from build123d import *

# Parameters (mm, degrees)
SKETCH_2_W          = 26.5
SKETCH_2_H          = 14.5
EXTRUDE_1_DEPTH     = 57
SKETCH_6_W          = 22.5
SKETCH_6_H          = 10.5
CUT_EXTRUDE_1_DEPTH = 49
SKETCH_7_W          = 26.5
SKETCH_7_H          = 16
EXTRUDE_2_DEPTH     = 24.8
FILLET_1_R          = 5
FILLET_2_R          = 1
FILLET_4_R          = 1
FILLET_5_R          = 1
FILLET_6_R          = 1
CUT_EXTRUDE_2_DEPTH = 20
SKETCH_10_W         = 10
SKETCH_10_H         = 3.5
CUT_EXTRUDE_3_DEPTH = 40


with BuildPart() as part:
    # ｽｹｯﾁ2 → ﾎﾞｽ - 押し出し1 (new body)
    with BuildSketch(Plane.XY):
        with Locations((13.25, 7.25)):
            Rectangle(SKETCH_2_W, SKETCH_2_H)
    extrude(amount=EXTRUDE_1_DEPTH)

    # ｽｹｯﾁ6 → ｶｯﾄ - 押し出し1 (cut)
    with BuildSketch(Plane.XY.offset(57)):
        with Locations((13.25, 7.25)):
            Rectangle(SKETCH_6_W, SKETCH_6_H)
    extrude(amount=-CUT_EXTRUDE_1_DEPTH, mode=Mode.SUBTRACT)

    # ｽｹｯﾁ7 → ﾎﾞｽ - 押し出し2 (add)
    with BuildSketch(Plane.XZ):
        with Locations((13.25, 8)):
            Rectangle(SKETCH_7_W, SKETCH_7_H)
    extrude(amount=EXTRUDE_2_DEPTH)

    # ﾌｨﾚｯﾄ1
    fillet_1_edges = [part.edges().sort_by_distance(p)[0] for p in [
        (13.25, 0, 16),
    ]]
    fillet(fillet_1_edges, radius=FILLET_1_R)

    # ﾌｨﾚｯﾄ2
    fillet_2_edges = [part.edges().sort_by_distance(p)[0] for p in [
        (26.5, 14.5, 28.5),
    ]]
    fillet(fillet_2_edges, radius=FILLET_2_R)

    # ﾌｨﾚｯﾄ4
    fillet_4_edges = [part.edges().sort_by_distance(p)[0] for p in [
        (26.5, -14.9, 16),
        (26.5, -24.8, 8),
        (26.5, -1.464466094, 17.464466094),
        (12.75, 14.5, 0),
        (26.207106781, 14.207106781, 0),
        (26.5, -5.65, 0),
        (26.5, 0, 39),
    ]]
    fillet(fillet_4_edges, radius=FILLET_4_R)

    # ﾌｨﾚｯﾄ5
    # the kernel refuses this fillet: 1 mm, written as the material it takes off along each edge
    with BuildSketch(Plane(origin=(25.5, -23.8, 15), x_dir=(0, -1, 0), z_dir=(0, 0, 1))) as fillet_5_piece_1_section:
        Polygon((0, 0), (FILLET_5_R, 0), (FILLET_5_R, FILLET_5_R), (0, FILLET_5_R), align=None)
    fillet_5_piece_1 = extrude(amount=FILLET_5_R, mode=Mode.PRIVATE)
    fillet_5_piece_1 = fillet_5_piece_1 - Plane(origin=(25.5, -23.8, 15), x_dir=(-0.7071067811865475, 0.7071067811865475, 0), z_dir=(0, 0, 1)) * Sphere(FILLET_5_R, mode=Mode.PRIVATE)
    add(fillet_5_piece_1, mode=Mode.SUBTRACT)
    with BuildSketch(Plane(origin=(25.5, -23.8, 1), x_dir=(0, -1, 0), z_dir=(0, 0, -1))) as fillet_5_piece_2_section:
        Polygon((0, 0), (FILLET_5_R, 0), (FILLET_5_R, -FILLET_5_R), (0, -FILLET_5_R), align=None)
    fillet_5_piece_2 = extrude(amount=FILLET_5_R, mode=Mode.PRIVATE)
    fillet_5_piece_2 = fillet_5_piece_2 - Plane(origin=(25.5, -23.8, 1), x_dir=(-0.7071067811865475, 0.7071067811865475, 0), z_dir=(0, 0, -1)) * Sphere(FILLET_5_R, mode=Mode.PRIVATE)
    add(fillet_5_piece_2, mode=Mode.SUBTRACT)
    with BuildSketch(Plane(origin=(1, -23.8, 15), x_dir=(-1, 0, 0), z_dir=(0, -1, 0))) as fillet_5_piece_3_section:
        Polygon((0, 0), (FILLET_5_R, 0), (FILLET_5_R, -FILLET_5_R), (0, -FILLET_5_R), align=None)
    fillet_5_piece_3 = extrude(amount=FILLET_5_R, mode=Mode.PRIVATE)
    fillet_5_piece_3 = fillet_5_piece_3 - Plane(origin=(1, -23.8, 15), x_dir=(0.7071067811865475, 0, -0.7071067811865475), z_dir=(0, -1, 0)) * Sphere(FILLET_5_R, mode=Mode.PRIVATE)
    add(fillet_5_piece_3, mode=Mode.SUBTRACT)
    with BuildSketch(Plane(origin=(1, -23.8, 1), x_dir=(-1, 0, 0), z_dir=(0, 0, -1))) as fillet_5_piece_4_section:
        Polygon((0, 0), (FILLET_5_R, 0), (FILLET_5_R, -FILLET_5_R), (0, -FILLET_5_R), align=None)
    fillet_5_piece_4 = extrude(amount=FILLET_5_R, mode=Mode.PRIVATE)
    fillet_5_piece_4 = fillet_5_piece_4 - Plane(origin=(1, -23.8, 1), x_dir=(0.7071067811865475, 0.7071067811865475, 0), z_dir=(0, 0, -1)) * Sphere(FILLET_5_R, mode=Mode.PRIVATE)
    add(fillet_5_piece_4, mode=Mode.SUBTRACT)
    with BuildSketch(Plane(origin=(0, -5, 16), x_dir=(0, 0, -1), z_dir=(0, -1, 0))) as fillet_5_piece_5:
        with BuildLine():
            CenterArc((FILLET_5_R, FILLET_5_R), FILLET_5_R, 180, 90)
            Line((0, FILLET_5_R), (0, 0))
            Line((0, 0), (FILLET_5_R, 0))
        make_face()
    extrude(amount=18.8, mode=Mode.SUBTRACT)
    with BuildSketch(Plane(origin=(0, -24.8, 15), x_dir=(0, 1, 0), z_dir=(0, 0, -1))) as fillet_5_piece_6:
        with BuildLine():
            CenterArc((FILLET_5_R, FILLET_5_R), FILLET_5_R, 180, 90)
            Line((0, FILLET_5_R), (0, 0))
            Line((0, 0), (FILLET_5_R, 0))
        make_face()
    extrude(amount=14, mode=Mode.SUBTRACT)
    with BuildSketch(Plane(origin=(1, -24.8, 0), x_dir=(0, 1, 0), z_dir=(1, 0, 0)), Plane(origin=(25.5, -24.8, 16), x_dir=(0, 1, 0), z_dir=(-1, 0, 0))) as fillet_5_piece_7:
        with BuildLine():
            CenterArc((FILLET_5_R, FILLET_5_R), FILLET_5_R, 180, 90)
            Line((0, FILLET_5_R), (0, 0))
            Line((0, 0), (FILLET_5_R, 0))
        make_face()
    extrude(amount=24.5, mode=Mode.SUBTRACT)
    with BuildSketch(Plane(origin=(0, -5, 21), x_dir=(0, 1, 0), z_dir=(0, 0, 1))) as fillet_5_piece_8:
        with BuildLine():
            CenterArc((5 + FILLET_5_R, -FILLET_5_R), FILLET_5_R, 90, 90)
            Line((5, -FILLET_5_R), (5, 0))
            Line((5, 0), (5 + FILLET_5_R, 0))
        make_face()
    revolve(axis=Axis((0, -5, 21), (-1, 0, 0)), revolution_arc=90, mode=Mode.SUBTRACT)
    with BuildSketch(Plane(origin=(0, 13.5, 0), x_dir=(0, 0, 1), z_dir=(0, -1, 0))) as fillet_5_piece_9:
        with BuildLine():
            CenterArc((FILLET_5_R, -FILLET_5_R), FILLET_5_R, 90, 90)
            Line((0, -FILLET_5_R), (0, 0))
            Line((0, 0), (FILLET_5_R, 0))
        make_face()
    extrude(amount=37.3, mode=Mode.SUBTRACT)
    with BuildSketch(Plane(origin=(0, 13.5, 1), x_dir=(0, 0, -1), z_dir=(0, -1, 0))) as fillet_5_piece_10:
        with BuildLine():
            CenterArc((1 - FILLET_5_R, FILLET_5_R), FILLET_5_R, 270, 90)
            Line((1, FILLET_5_R), (1, 0))
            Line((1, 0), (1 - FILLET_5_R, 0))
        make_face()
    revolve(axis=Axis((0, 13.5, 1), (1, 0, 0)), revolution_arc=90, mode=Mode.SUBTRACT)
    with BuildSketch(Plane(origin=(0, 14.5, 1), x_dir=(1, 0, 0), z_dir=(0, 0, 1))) as fillet_5_piece_11:
        with BuildLine():
            CenterArc((FILLET_5_R, -FILLET_5_R), FILLET_5_R, 90, 90)
            Line((0, -FILLET_5_R), (0, 0))
            Line((0, 0), (FILLET_5_R, 0))
        make_face()
    extrude(amount=58.5, mode=Mode.SUBTRACT)
    with BuildSketch(Plane(origin=(0, 0, 21), x_dir=(1, 0, 0), z_dir=(0, 0, 1))) as fillet_5_piece_12:
        with BuildLine():
            CenterArc((FILLET_5_R, FILLET_5_R), FILLET_5_R, 180, 90)
            Line((0, FILLET_5_R), (0, 0))
            Line((0, 0), (FILLET_5_R, 0))
        make_face()
    extrude(amount=38.5, mode=Mode.SUBTRACT)

    # ﾌｨﾚｯﾄ6
    fillet_6_edges = [part.edges().sort_by_distance(p)[0] for p in [
        (13.25, 14.5, 57),
        (26.207106781, 14.207106781, 57),
        (26.5, 7.25, 57),
        (26.207106781, 0.292893219, 57),
        (0, 7.25, 57),
        (13.25, 0, 57),
        (0.292893219, 0.292893219, 57),
        (0.292893219, 14.207106781, 57),
    ]]
    fillet(fillet_6_edges, radius=FILLET_6_R)

    # ｽｹｯﾁ8 → ｶｯﾄ - 押し出し2 (cut)
    with BuildSketch(Plane.XZ.offset(24.8)):
        Polygon((9.75, 16), (16.75, 16), (16.75, 6.5), (15.25, 6.5), (15.25, 5.5), (18.25, 5.5), (18.25, 2), (8.25, 2), (8.25, 5.5), (11.25, 5.5), (11.25, 6.5), (9.75, 6.5), align=None)
    extrude(amount=-CUT_EXTRUDE_2_DEPTH, mode=Mode.SUBTRACT)

    # ｽｹｯﾁ10 → ｶｯﾄ - 押し出し3 (cut)
    with BuildSketch(Plane.XZ.offset(24.8)):
        with Locations((13.25, 3.75)):
            Rectangle(SKETCH_10_W, SKETCH_10_H)
    extrude(amount=-CUT_EXTRUDE_3_DEPTH, mode=Mode.SUBTRACT)


solid = part.part
Here's how the part is built. I have some questions about the finished solid (model axes, mm). A direction names the side the tool comes from. Coordinates: 2 decimals unless noted, no trailing zeros. Loops run counter-clockwise (first coordinate to the right, second up) from the corner with the lowest first, then second, coordinate; pieces in that order, holes last.
1. Imagine slicing it at A-A, the plane z = 36. Please give me the cut outline in (x, y), and give its area (3 significant figures).
2. For faces 4 (the flat face through (13, 14.5, 28)), 5 (the flat face through (13, 12.5, 33)), 6 (the flat face through (5, -14, 16)), 7 (the flat face through (13, -1, 5.5)), which set-ups out of +Z, -Z, +X, -X, +Y, -Y let a thin tool reach every point of the face, with its end or its side?
3. Imagine slicing it at B-B, the plane y = -10. Please give me the cut outline in (x, z), and give its area (3 significant figures).
4. Imagine slicing it at C-C, the plane x = 7.5. Please give me the cut outline in (y, z), and give its area (3 significant figures).
5. For P1, Ø1.2, axis at x = 16.5, y = -10.5, coming from the +Z side; P2, Ø5, axis at x = 14.5, y = 9, coming from the +Z side; P3, Ø5, axis at x = 15.5, z = 42, coming from the -Y side, each with a flat end and sliding along its axis, tell me the tip position at first contact or that it passes through.
6. Imagine slicing it at D-D, the plane y = 4.5. Please give me the cut outline in (x, z).
7. If we mould it in two halves opening along X, with no side actions, what happens to faces 1 (the flat face through (21, -14, 16)), 2 (the flat face through (13, 7, 8)), 3 (the flat face through (0, 3, 22))? For each: pulls with the +X half, pulls with the -X half, needs draft (parallel to the pull), parting line crosses it, or undercut.
8. I need wall thicknesses on L1, parallel to Y at x = 17.25, z = 9; L2, parallel to Y at x = 8, z = 22; L3, parallel to Z at x = 14.5, y = 10. Which ranges of each line are inside material? Lowest first, please.
Taken from the geometry:
1. outline: (0, 1) arc R1 ccw to (1, 0) - (25.5, 0) arc R1 ccw to (26.5, 1) - (26.5, 13.5) arc R1 ccw to (25.5, 14.5) - (1, 14.5) arc R1 ccw to (0, 13.5) - close; hole (2, 2) - (24.5, 2) - (24.5, 12.5) - (2, 12.5) - close
1. area: 147 mm2
2. face 4: +Z, -Z, +X, -X, +Y
2. face 5: +Z
2. face 6: +Z, +X, -X, -Y
2. face 7: +Y, -Y
3. outline: (0, 1) arc R1 ccw to (1, 0) - (25.5, 0) arc R1 ccw to (26.5, 1) - (26.5, 15) arc R1 ccw to (25.5, 16) - (16.75, 16) - (16.75, 6.5) - (15.25, 6.5) - (15.25, 5.5) - (18.25, 5.5) - (18.25, 2) - (8.25, 2) - (8.25, 5.5) - (11.25, 5.5) - (11.25, 6.5) - (9.75, 6.5) - (9.75, 16) - (1, 16) arc R1 ccw to (0, 15) - close
3. area: 318 mm2
4. outline: (-24.8, 1) arc R1 ccw to (-23.8, 0) - (13.5, 0) arc R1 ccw to (14.5, 1) - (14.5, 56) arc R1 ccw to (13.5, 57) - (12.5, 57) - (12.5, 8) - (2, 8) - (2, 57) - (1, 57) arc R1 ccw to (0, 56) - (0, 21) arc R5 cw to (-5, 16) - (-23.8, 16) arc R1 ccw to (-24.8, 15) - close
4. area: 713 mm2
5. P1: stops at z = 16
5. P2: stops at z = 8
5. P3: stops at y = 0
6. outline: (0, 1) arc R1 ccw to (1, 0) - (25.5, 0) arc R1 ccw to (26.5, 1) - (26.5, 56) arc R1 ccw to (25.5, 57) - (24.5, 57) - (24.5, 8) - (2, 8) - (2, 57) - (1, 57) arc R1 ccw to (0, 56) - close; hole (8.25, 2) - (18.25, 2) - (18.25, 5.5) - (8.25, 5.5) - close
7. face 1: needs draft
7. face 2: undercut
7. face 3: pulls with the -X half
8. L1: y = -24.8 to 2, 12.5 to 14.5
8. L2: y = 0 to 2, 12.5 to 14.5
8. L3: z = 0 to 2, 5.5 to 8
